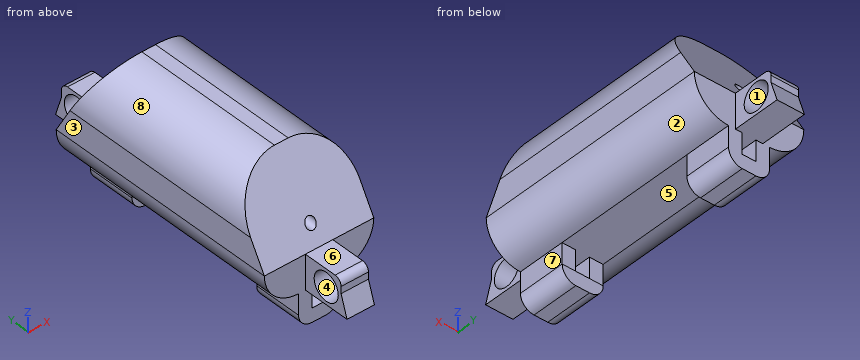
Autodesk Inventor part; units mm, degrees
ref_plane "YZ Plane" through (0, 0, 0) normal (1, 0, 0) x (0, 1, 0)
ref_plane "XZ Plane" through (0, 0, 0) normal (0, 1, 0) x (-1, 0, 0)
ref_plane "XY Plane" through (0, 0, 0) normal (0, 0, 1) x (1, 0, 0)
sketch "Sketch3" plane through (0, 0, 0) normal (0, 0, 1) x (1, 0, 0)
  line L0 (0, 0) -> (16, 0)
  line L1 (16, 0) -> (16, 35)
  line L2 (16, 35) -> (0, 35)
  line L3 (0, 35) -> (0, 0)
  dimension "d0" = 16
  dimension "d1" = 35
extrude "Extrusion1" add sketch "Sketch3" along normal blind 16
fillet "Fillet1" radius 7 2 edges at (16, 17.5, 16) (0, 17.5, 16)
fillet "Fillet2" radius 5 2 edges at (16, 17.5, 0) (0, 17.5, 0)
sketch "Sketch4" plane through (16, 0, 9) normal (1, 0, 0) x (0, 0, -1)
  line L0 (4, 35) -> (0, 35)
  line L1 (4, 35) -> (-7, 28.6491)
  line L2 (-7, 35) -> (-7, 0)
  line L3 (4, 35) -> (16.7017, 35) construction
  line L4 (-7, 28.6491) -> (-7, 35)
  line L5 (-7, 35) -> (4, 35)
  line L6 (4, 0) -> (0, 0)
  line L7 (4, 0) -> (-7, 6.3509)
  line L8 (4, 0) -> (16.7017, 0) construction
  line L9 (-7, 6.3509) -> (-7, 0)
  line L10 (-7, 0) -> (4, 0)
  point P0 (9, 0)
  point P1 (-7, 0)
  point P2 (0, 0)
  dimension "d6" = 150
  dimension "d7" = 150
extrude "Extrusion2" cut sketch "Sketch4" against normal through all
sketch "Sketch5" plane through (5, 35, 0) normal (0, 1, 0) x (1, 0, 0)
  line L0 (-5, -9) -> (-5, -5)
  line L1 (0, 0) -> (6, 0)
  line L2 (5, 0) -> (1, 0)
  line L3 (1, 0) -> (1, -5)
  line L4 (1, -5) -> (5, -5)
  line L5 (5, -5) -> (5, 0)
  line L6 (1, 0) -> (5, 0)
  point P0 (-5, 0)
  dimension "d47" = 4
extrude "Extrusion3" add sketch "Sketch5" along normal blind 6
sketch "Sketch11" plane through (0, 0, 0) normal (0, 0, -1) x (-1, 0, 0)
  line L0 (-11, 0) -> (-11, 35)
  line L1 (-9, 28.6491) -> (-9, 6.3509)
  line L2 (-11, 0) -> (-9, 0)
  line L3 (-9, 0) -> (-9, 7)
  line L4 (-9, 7) -> (-11, 7)
  line L5 (-11, 7) -> (-11, 0)
  line L6 (-5, 0) -> (-7, 0)
  line L7 (-7, 0) -> (-7, 7)
  line L8 (-7, 7) -> (-5, 7)
  line L9 (-5, 7) -> (-5, 0)
  line L10 (-11, 35) -> (-9, 35)
  line L11 (-9, 35) -> (-9, 28)
  line L12 (-9, 28) -> (-11, 28)
  line L13 (-11, 28) -> (-11, 35)
  line L14 (-5, 35) -> (-7, 35)
  line L15 (-7, 35) -> (-7, 28)
  line L16 (-7, 28) -> (-5, 28)
  line L17 (-5, 28) -> (-5, 35)
  point P0 (0, 0)
  point P1 (-9, 6.3509)
  point P2 (-11, 28)
  dimension "d32" = 7
  dimension "d33" = 2
  dimension "d34" = 7
  dimension "d35" = 7
  dimension "d36" = 7
extrude "Extrusion9" add sketch "Sketch11" along normal blind 3 contours L0 L4 L1 L3 L2 | L0 L10 L11 L1 L12 | L6 L7 L8 L9 | L17 L16 L15 L14
sketch "Sketch12" plane through (0, 0, -3) normal (0, 0, -1) x (-1, 0, 0)
  line L0 (-9, 35) -> (-11, 35)
  line L1 (-5, 28) -> (-7, 28)
  line L2 (-11, 35) -> (-5, 35)
  line L3 (-5, 35) -> (-5, 28)
  line L4 (-5, 28) -> (-11, 28)
  line L5 (-11, 28) -> (-11, 35)
  line L6 (-11, 0) -> (-16, 0)
  line L7 (-11, 0) -> (-5, 0)
  line L8 (-5, 0) -> (-5, 7.0241)
  line L9 (-5, 7.0241) -> (-11, 7.0241)
  line L10 (-11, 7.0241) -> (-11, 0)
  point P0 (0, 0)
  point P1 (-5, -5)
  point P2 (-11, 2)
extrude "Extrusion10" add sketch "Sketch12" along normal blind 2
sketch "Sketch13" plane through (0, 0, 5) normal (0, -1, 0) x (1, 0, 0)
  circle A0 centre (8, 2.5) radius 0.75
  point P0 (0, -5)
  dimension "d42" = 1.5
extrude "Extrusion11" cut sketch "Sketch13" against normal through all
fillet "Fillet4" radius 2 4 edges at (11, 31.5, -5) (5, 31.5, -5) (5, 3.5121, -5) (11, 3.5121, -5)
sketch "Sketch14" plane through (10, 35, 5) normal (1, 0, 0) x (0, 0, -1)
  circle A0 centre (2.5, 3.5) radius 2.025
  line L0 (0, 6) -> (5, 6)
  point P0 (5, -35)
  dimension "d48" = 4.05
  dimension "d59" = 2.5
extrude "Extrusion12" cut sketch "Sketch14" against normal blind 5
sketch "Sketch15" plane through (0, 0, 5) normal (0, -1, 0) x (1, 0, 0)
  line L0 (10, -5) -> (10, 0)
  line L1 (10, 0) -> (6, 0)
  line L2 (6, 0) -> (6, -5)
  line L3 (6, -5) -> (10, -5)
  line L4 (10, -5) -> (10, 0)
  point P0 (0, -5)
  point P1 (10, -0.475)
  point P2 (6, -0.475)
  dimension "d60" = 5
  dimension "d61" = 4
extrude "Extrusion13" add sketch "Sketch15" along normal blind 6
sketch "Sketch16" plane through (10, 0, 5) normal (1, 0, 0) x (0, 0, -1)
  circle A0 centre (2.5, -3.5) radius 2.025
  line L0 (5, -6) -> (0, -6)
  point P0 (5, 0)
  dimension "d54" = 4.05
  dimension "d58" = 2.5
extrude "Extrusion14" cut sketch "Sketch16" against normal blind 5
fillet "Fillet7" radius 1 1 edges at (8, -6, 5)
sketch "Sketch17" plane through (0, -6, 5) normal (0, -1, 0) x (1, 0, 0)
  line L0 (6, -5) -> (10, -5)
  line L1 (6, -4.525) -> (6, -0.475)
  line L2 (10, -5) -> (6, -5)
  line L3 (6, -5) -> (6, -2)
  line L4 (6, -2) -> (10, -2)
  line L5 (10, -2) -> (10, -5)
  point P0 (0, -5)
  dimension "d63" = 3
extrude "Extrusion15" add sketch "Sketch17" along normal blind 1
fillet "Fillet8" radius 1 1 edges at (8, 41, 5)
sketch "Sketch18" plane through (5, 41, 0) normal (0, 1, 0) x (1, 0, 0)
  line L0 (1, -3) -> (5, -3)
  line L1 (1, -5) -> (1, 0)
  line L2 (5, -3) -> (1, -3)
  line L3 (1, -3) -> (1, 0)
  line L4 (1, 0) -> (5, 0)
  line L5 (5, 0) -> (5, -3)
  point P0 (-5, 0)
extrude "Extrusion16" add sketch "Sketch18" along normal blind 1
sketch "Sketch19" plane through (6, 0, 0) normal (-1, 0, 0) x (0, 0, 1)
  line L0 (3, -6) -> (3, -7)
  line L1 (0, 0) -> (0, -7)
  line L2 (3, -6) -> (0, -7)
  line L3 (0, -7) -> (3, -7)
  line L4 (3, -7) -> (3, -6)
extrude "Extrusion17" cut sketch "Sketch19" against normal through all
sketch "Sketch20" plane through (6, 35, 0) normal (-1, 0, 0) x (0, 0, 1)
  line L0 (4, 6) -> (3, 6)
  line L1 (0, 0) -> (0, 7)
  line L2 (3, 6) -> (0, 7)
  line L3 (0, 7) -> (3, 7)
  line L4 (3, 7) -> (3, 6)
  point P0 (0, -35)
extrude "Extrusion18" cut sketch "Sketch20" against normal through all
properties part number "FingerMiddle"
Source: CAD feature listing. Evaluate the final solid. Frame: model axes, mm. Face numbers are marked on the shaded views. A direction names the side the tool comes from. Give positions to 0.01 mm unless a question says otherwise; leave off trailing zeros. Write each loop counter-clockwise with the first axis right and the second up, starting at its lowest first coordinate (ties: lowest second). Pieces come first, ordered by that corner, then holes. Notation, with made-up numbers: M -1,48.25 L 26,48.25 A18 cw 26,63.25 Z; hole C 58.25,-20.5 d8. An arc over 180 degrees is marked long. Return JSON: item names as keys, results as strings. Group by question number.
1) Pull-direction query (Z, two-part tool) for the marked faces 1, 2 and 3; classes: pulls with the +Z half, pulls with the -Z half, needs draft (parallel to the pull), parting line crosses it, or undercut.
2) Cut plane D-D, the plane z = 2.5. Output: boundary loops of the cut face in (x, y) (3 decimals).
3) Cut plane A-A, the plane y = 38.5. Output: boundary loops of the cut face in (x, z) (3 decimals).
4) Cut plane B-B, the plane y = 23.5. Output: boundary loops of the cut face in (x, z), plus the area to 3 significant figures.
5) Material intervals for line 1 along Y through (x, z) = (8.1, 2.5) (3 decimals); line 2 along Z through (x, y) = (8, 18.5); line 3 along Y through (x, z) = (6.75, 4), sorted ascending. Write a range as [from, to].
6) Cut plane C-C, the plane x = 8. Output: boundary loops of the cut face in (y, z) (3 decimals).
7) Set-up query: the marked faces 4, 5, 6, 7 and 8. Return all of +Z, -Z, +X, -X, +Y, -Y with unobstructed straight access to the full face (end or side cutting, diameter ignored); none if empty.
8) Pin query (flat end, axial travel): P1, Ø0.9, axis at y = 32, z = -2, coming from the -X side; P2, Ø2, axis at x = 8, y = 30.5, coming from the +Z side; P3, Ø8, axis at y = 20.5, z = -2.5, coming from the +X side. Return the tip coordinate at first contact, or that it passes through.
Recorded:
{
 "1": {"face 1": "undercut", "face 2": "pulls with the -Z half", "face 3": "needs draft"},
 "2": {"outline": "M 0.67,0 L 6,0 L 6,-1.475 L 10,-1.475 L 10,0 L 15.33,0 L 15.33,35 L 10,35 L 10,36.475 L 6,36.475 L 6,35 L 0.67,35 Z; M 6,-6.167 L 10,-6.167 L 10,-5.525 L 6,-5.525 Z; M 6,40.525 L 10,40.525 L 10,41.167 L 6,41.167 Z"},
 "3": {"outline": "M 6,0 L 10,0 L 10,0.475 L 6,0.475 Z; M 6,4.525 L 10,4.525 L 10,5 L 6,5 Z"},
 "4": {"outline": "M 0,5 A5 ccw 5,0 L 11,0 A5 ccw 16,5 L 16,9 A7 ccw 9,16 L 7,16 A7 ccw 0,9 Z; hole C 8,7.5 d1.5", "area": "222 mm²"},
 "5": {"line 1": "y = [-6.167, -5.525], [-1.475, 36.475], [40.525, 41.167]", "line 2": "z = [0, 6.75], [8.25, 16]", "line 3": "y = [-6, -4.86], [-2.14, 37.14], [39.86, 41]"},
 "6": {"outline": "M -7,0 L 42,0 L 41,3 L 41,4 A1 ccw 40,5 L 35,5 L 33.99,6.75 L 1.01,6.75 L 0,5 L -5,5 A1 ccw -6,4 L -6,3 Z; M 0,-5 L 7.024,-5 L 7.024,-3 L 0,-3 Z; M 1.876,8.25 L 33.124,8.25 L 28.649,16 L 6.351,16 Z; M 28,-5 L 35,-5 L 35,-3 L 28,-3 Z; hole C -3.5,2.5 d4.05; hole C 38.5,2.5 d4.05"},
 "7": {"face 4": "+X, -X", "face 5": "none", "face 6": "+Z, +X, -X, -Y", "face 7": "-Z, +X, +Y, -Y", "face 8": "+Z, -X, +Y, -Y"},
 "8": {"P1": "stops at x = 5", "P2": "stops at z = 14.53", "P3": "stops at x = 14.57"}
}
